Input: part model. Units: mm. Frame: model coordinates. Face numbers are marked on the shaded views. A direction names the side the tool comes from. Give positions to 0.01 mm unless a question says otherwise; leave off trailing zeros. Loops run counter-clockwise (first coordinate to the right, second up) from the corner with the lowest first, then second, coordinate; pieces in that order, holes last. Notation, with made-up numbers: M 69.25,13.5 L 82.25,13.5 A20 cw 82.25,39.5 Z; hole C 12,54.25 d4. An arc over 180 degrees is marked long. Answer as a JSON object with one key per item and string values. Group by question number.
1) Section query C-C on x = -14. Return loops of the section in (y, z).
2) Ray query, L1, parallel to Z at x = -22.5, y = 4; L2, parallel to Y at x = 1, z = -48.5; L3, parallel to X at y = -26, z = -16. Return the intervals inside material, ascending.
3) Draft query along Z for the marked faces 4, 5 and 6. Return one class per face: +Z half, -Z half, draft (parallel to the pull), parting line (faces both ways), or undercut.
4) Access query for the marked faces 1, 2 and 3. Directions: +Z, -Z, +X, -X, +Y, -Y. A direction counts if a zero-diameter tool reaches every point of the face in a straight line with its end or side. Return the directions, or none.
5) First-contact query: P1, Ø12, axis at y = 13.5, z = -142.5, coming from the -X side; P2, Ø4, axis at x = 34.5, y = -12.5, coming from the -Z side; P3, Ø14, axis at x = 32.5, y = -12.5, coming from the +Z side; P4, Ø7.5, axis at y = 0, z = -12.7, coming from the +X side. Flat tips, straight axial feed; report the tip coordinate or a pass-through.
6) Section query B-B on z = -215.9. Return loops of the section in (x, y), plus the area to 3 significant figures.
7) Section query D-D on y = 25.5. Return loops of the section in (x, z), plus the area to 3 significant figures.
8) Section query A-A on y = 0. Return loops of the section in (x, z).
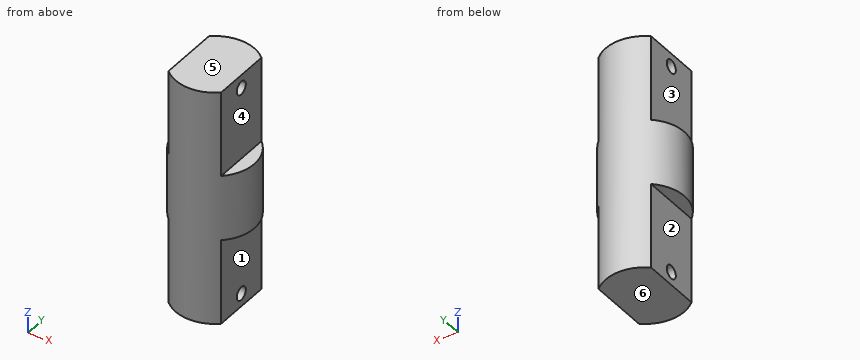
from build123d import *

# Parameters (mm, degrees)
SKETCH2_R           = 38.1
BOSS_EXTRUDE1_DEPTH = 228.6
CUT_EXTRUDE1_START  = 25.4
SKETCH3_W           = 165.1
SKETCH3_H           = 76.2
CUT_EXTRUDE1_DEPTH  = 25.4
CUT_EXTRUDE2_START  = -25.4
SKETCH3_2_W         = 165.1
SKETCH3_2_H         = 76.2
CUT_EXTRUDE2_DEPTH  = 25.4
CUT_EXTRUDE3_REACH  = 242.295
SKETCH4_R           = 6.35


with BuildPart() as part:
    # Sketch2 → Boss-Extrude1 (new body)
    with BuildSketch(Plane.XY):
        Circle(SKETCH2_R)
    extrude(amount=-BOSS_EXTRUDE1_DEPTH)

    # Sketch3 → Cut-Extrude1 (cut)
    with BuildSketch(Plane(origin=(0, 0, 0), x_dir=(0, 0, -1), z_dir=(1, 0, 0)).offset(CUT_EXTRUDE1_START)):
        Rectangle(SKETCH3_W, SKETCH3_H)
    cut_extrude1 = extrude(amount=CUT_EXTRUDE1_DEPTH, mode=Mode.SUBTRACT)

    # Sketch3<2> → Cut-Extrude2 (cut)
    with BuildSketch(Plane(origin=(0, 0, 0), x_dir=(0, 0, -1), z_dir=(1, 0, 0)).offset(CUT_EXTRUDE2_START)):
        Rectangle(SKETCH3_2_W, SKETCH3_2_H)
    cut_extrude2 = extrude(amount=-CUT_EXTRUDE2_DEPTH, mode=Mode.SUBTRACT)

    # Sketch4 → Cut-Extrude3 (cut, up to next)
    with BuildSketch(Plane(origin=(25.4, 0, 0), x_dir=(0, 0, -1), z_dir=(1, 0, 0)), mode=Mode.PRIVATE) as cut_extrude3_sk1:
        with Locations((12.7, 0)):
            Circle(SKETCH4_R)
    cut_extrude3_tool1 = extrude(cut_extrude3_sk1.sketch, amount=-CUT_EXTRUDE3_REACH, mode=Mode.PRIVATE) & part.part
    cut_extrude3 = cut_extrude3_tool1.solids().sort_by_distance((25.4, 0, -12.7))[0]
    add(cut_extrude3, mode=Mode.SUBTRACT)

    # Mirror1: Cut-Extrude1, Cut-Extrude2, Cut-Extrude3 across plane
    add(cut_extrude1.mirror(Plane.XY.offset(-114.3)), mode=Mode.SUBTRACT)
    add(cut_extrude2.mirror(Plane.XY.offset(-114.3)), mode=Mode.SUBTRACT)
    add(cut_extrude3.mirror(Plane.XY.offset(-114.3)), mode=Mode.SUBTRACT)


solid = part.part
Output:
{
 "1": {"outline": "M -35.43,-228.6 L 35.43,-228.6 L 35.43,0 L -35.43,0 Z; hole C 0,-215.9 d12.7; hole C 0,-12.7 d12.7"},
 "2": {"L1": "z = -228.6 to -220.83, -210.97 to -17.63, -7.77 to 0", "L2": "y = -38.09 to 38.09", "L3": "x = -25.4 to 25.4"},
 "3": {"face 4": "draft", "face 5": "+Z half", "face 6": "-Z half"},
 "4": {"face 1": "-Z, +X, +Y, -Y", "face 2": "-Z, -X, +Y, -Y", "face 3": "+Z, -X, +Y, -Y"},
 "5": {"P1": "stops at x = -37.35", "P2": "stops at z = -146.05", "P3": "stops at z = -82.55", "P4": "passes through"},
 "6": {"outline": "M -25.4,-28.4 A38.1 ccw 25.4,-28.4 L 25.4,-6.35 L -25.4,-6.35 Z; M -25.4,6.35 L 25.4,6.35 L 25.4,28.4 A38.1 ccw -25.4,28.4 Z", "area": "2,920 mm^2"},
 "7": {"outline": "M -28.31,-146.05 L -25.4,-146.05 L -25.4,-228.6 L 25.4,-228.6 L 25.4,-146.05 L 28.31,-146.05 L 28.31,-82.55 L 25.4,-82.55 L 25.4,0 L -25.4,0 L -25.4,-82.55 L -28.31,-82.55 Z", "area": "12,000 mm^2"},
 "8": {"outline": "M -38.1,-146.05 L -25.4,-146.05 L -25.4,-209.55 L 25.4,-209.55 L 25.4,-146.05 L 38.1,-146.05 L 38.1,-82.55 L 25.4,-82.55 L 25.4,-19.05 L -25.4,-19.05 L -25.4,-82.55 L -38.1,-82.55 Z; M -25.4,-228.6 L 25.4,-228.6 L 25.4,-222.25 L -25.4,-222.25 Z; M -25.4,-6.35 L 25.4,-6.35 L 25.4,0 L -25.4,0 Z"}
}
